from build123d import *

# Parameters (mm, degrees)
F0_W          = 70
F0_H          = 16
F1_DEPTH      = 22
F1_DEPTH_BACK = 22
F2_DEPTH      = 10
F2_DEPTH_BACK = 10
F3_R          = 21.99999


# Not quite as in the source:
# - a fillet or chamfer is up to 0.001 mm smaller than in the source, because OpenCascade refuses the exact size


with BuildPart() as f1:
    # F0 (on Front) → F1 (new body, two sides)
    with BuildSketch(Plane.XZ) as f1_sk:
        with BuildLine():
            Line((24, 0), (10, 0))
            ThreePointArc((10, 0), (0, -10), (-10, 0))
            Line((-10, 0), (-24, 0))
            ThreePointArc((-24, 0), (-16.9705627485, -16.9705627485), (0, -24))
            ThreePointArc((0, -24), (16.9705627485, -16.9705627485), (24, 0))
        make_face()
        with BuildLine():
            ThreePointArc((-10, 0), (0, 10), (10, 0))
            Line((10, 0), (24, 0))
            ThreePointArc((24, 0), (0, 24), (-24, 0))
            Line((-24, 0), (-10, 0))
        make_face()
        with BuildLine():
            Line((24, -24), (24, 0))
            ThreePointArc((24, 0), (16.9705627485, -16.9705627485), (0, -24))
            Line((0, -24), (24, -24))
        make_face()
        with BuildLine():
            ThreePointArc((0, -24), (-16.9705627485, -16.9705627485), (-24, 0))
            Line((-24, 0), (-24, -24))
            Line((-24, -24), (0, -24))
        make_face()
        Polygon((24, -24), (0, -24), (-24, -24), (-24, -40), (24, -40), align=None)
        with Locations((59, -32)):
            Rectangle(F0_W, F0_H)
    extrude(amount=F1_DEPTH)
    extrude(f1_sk.sketch, amount=-F1_DEPTH_BACK)

    # F0 (on Front) → F2 (cut, two sides)
    with BuildSketch(Plane.XZ) as f2_sk:
        with BuildLine():
            ThreePointArc((-10, 0), (0, 10), (10, 0))
            Line((10, 0), (24, 0))
            ThreePointArc((24, 0), (0, 24), (-24, 0))
            Line((-24, 0), (-10, 0))
        make_face()
        with BuildLine():
            Line((24, -24), (24, 0))
            ThreePointArc((24, 0), (16.9705627485, -16.9705627485), (0, -24))
            Line((0, -24), (24, -24))
        make_face()
        with BuildLine():
            ThreePointArc((0, -24), (-16.9705627485, -16.9705627485), (-24, 0))
            Line((-24, 0), (-24, -24))
            Line((-24, -24), (0, -24))
        make_face()
        with BuildLine():
            Line((24, 0), (10, 0))
            ThreePointArc((10, 0), (0, -10), (-10, 0))
            Line((-10, 0), (-24, 0))
            ThreePointArc((-24, 0), (-16.9705627485, -16.9705627485), (0, -24))
            ThreePointArc((0, -24), (16.9705627485, -16.9705627485), (24, 0))
        make_face()
    extrude(amount=-F2_DEPTH, mode=Mode.SUBTRACT)
    extrude(f2_sk.sketch, amount=F2_DEPTH_BACK, mode=Mode.SUBTRACT)

    # F3 (radius 22 in the source; OpenCascade refuses exactly that, so slightly less here)
    f3_edges = [f1.edges().sort_by_distance(p)[0] for p in [
        (94, -22, -32),
        (94, 22, -32),
    ]]
    fillet(f3_edges, radius=F3_R)


solid = f1.part
Source: CAD feature listing. Evaluate the final solid. Frame: model axes, mm. A direction names the side the tool comes from. Give positions to 0.01 mm unless a question says otherwise; leave off trailing zeros. Write each loop counter-clockwise with the first axis right and the second up, starting at its lowest first coordinate (ties: lowest second). Pieces come first, ordered by that corner, then holes. Notation, with made-up numbers: M 9.25,4 L 23.25,4 A12 cw 23.25,11 Z; hole C 25,45 d10. An arc over 180 degrees is marked long. Return JSON: item names as keys, results as strings. Group by question number.
1) Cut plane C-C, the plane y = 12. Output: boundary loops of the cut face in (x, z).
2) Pin query (flat end, axial travel): P1, Ø9.5, axis at y = -14, z = -13, coming from the +X side. Return the tip coordinate at first contact, or that it passes through.
3) Cut plane A-A, the plane z = -19.5. Output: boundary loops of the cut face in (x, y).
4) Material intervals for line 1 along Z through (x, y) = (0, -16.5); line 2 along X through (y, z) = (-16, 0); line 3 along Y through (x, z) = (8, -23.5), sorted ascending. Write a range as [from, to].
5) Set-up query: faces 1 (the face through (-0.3, -10, -10.3)), 2 (the face through (24, 16, -12)), 3 (the face through (0.528, 15.916, 23.994)). Return all of +Z, -Z, +X, -X, +Y, -Y with unobstructed straight access to the full face (end or side cutting, diameter ignored); none if empty.
6) Cut plane B-B, the plane x = 0. Output: boundary loops of the cut face in (y, z), plus the area to 3 significant figures.
7) Pull-direction query (Y, two-part tool) for faces 4 (the face through (47, 0, -24)), 5 (the face through (-24, -0.3, -24.2)), 6 (the face through (13, -22, -15)), 7 (the face through (-0.3, 10, -10.3)); classes: pulls with the +Y half, pulls with the -Y half, needs draft (parallel to the pull), parting line crosses it, or undercut.
8) Cut plane D-D, the plane x = -16. Output: boundary loops of the cut face in (y, z), plus the area to 3 significant figures.
Recorded:
{
 "1": {"outline": "M -24,-40 L 90.44,-40 L 90.44,-24 L 24,-24 L 24,0 A24 ccw -24,0 Z; hole C 0,0 d20"},
 "2": {"P1": "stops at x = 24"},
 "3": {"outline": "M -24,-22 L 24,-22 L 24,-10 L -24,-10 Z; M -24,10 L 24,10 L 24,22 L -24,22 Z"},
 "4": {"line 1": "z = [-40, -10], [10, 24]", "line 2": "x = [-24, -10], [10, 24]", "line 3": "y = [-22, -10], [10, 22]"},
 "5": {"face 1": "+Z, +X, -X", "face 2": "+Z, +X, +Y, -Y", "face 3": "+Z, +Y, -Y"},
 "6": {"outline": "M -22,-40 L 22,-40 L 22,-10 L 10,-10 L 10,-24 L -10,-24 L -10,-10 L -22,-10 Z; M -22,10 L -10,10 L -10,24 L -22,24 Z; M 10,10 L 22,10 L 22,24 L 10,24 Z", "area": "1,380 mm²"},
 "7": {"face 4": "undercut", "face 5": "needs draft", "face 6": "pulls with the -Y half", "face 7": "undercut"},
 "8": {"outline": "M -22,-40 L 22,-40 L 22,17.89 L 10,17.89 L 10,-24 L -10,-24 L -10,17.89 L -22,17.89 Z", "area": "1,710 mm²"}
}
